Autodesk Inventor part; units mm, degrees
ref_plane "YZ Plane" through (0, 0, 0) normal (1, 0, 0) x (0, 1, 0)
ref_plane "XZ Plane" through (0, 0, 0) normal (0, 1, 0) x (-1, 0, 0)
ref_plane "XY Plane" through (0, 0, 0) normal (0, 0, 1) x (1, 0, 0)
sketch "Sketch1" plane through (0, 0, 0) normal (0, 0, 1) x (1, 0, 0)
  line L0 (-12.7, 25.4) -> (12.7, 25.4)
  line L1 (12.7, 25.4) -> (12.7, -25.4)
  line L2 (12.7, -25.4) -> (-12.7, -25.4)
  line L3 (-12.7, -25.4) -> (-12.7, 25.4)
  line L4 (-12.7, 25.4) -> (12.7, -25.4) construction
  line L5 (12.7, 25.4) -> (-12.7, -25.4) construction
  point P0 (0, 0)
  dimension "d0" = 25.4
  dimension "d1" = 50.8
extrude "Extrusion1" add sketch "Sketch1" along normal blind 1.397
sketch "Sketch3" plane through (12.7, -25.4, 0) normal (1, 0, 0) x (0, 0, -1)
  line L0 (0, 50.8) -> (0, 0)
  line L1 (0, 50.8) -> (-1.397, 50.8)
  line L2 (-1.397, 0) -> (-1.397, 50.8)
  line L3 (0, 0) -> (-1.397, 0)
  line L4 (-1.397, 0) -> (-1.905, 0)
  line L5 (-1.397, 0) -> (-1.397, 1.27)
  line L6 (-1.397, 53.34) -> (-1.397, 0)
  line L7 (-1.651, 1.27) -> (-1.397, 1.27)
  line L8 (-1.651, 1.27) -> (-1.905, 0)
  point P0 (0, 25.4)
  dimension "d8" = 0.508
  dimension "d9" = 1.27
  dimension "d10" = 0.254
ref_plane "Work Plane1" through (0, 0, 1.651) normal (0, 0, 1) x (1, 0, 0)
sketch "Sketch6" plane through (0, 0, 1.651) normal (0, 0, 1) x (1, 0, 0)
  line L0 (12.7, -24.13) -> (12.7, -25.4)
  line L1 (12.7, -25.4) -> (12.7, 25.4)
  line L2 (12.7, -24.765) -> (-12.7, -24.765)
  line L3 (-12.7, -25.4) -> (12.7, -25.4)
  line L4 (-12.7, -25.4) -> (12.7, -25.4)
  point P0 (0, 0)
  dimension "d12" = 0.635
sweep "Sweep1" add profiles "Sketch3" path "Sketch6" path curves L2 contours L4 L8 L7 L2
ref_plane "Work Plane2" through (-12.7, 0, 0) normal (0, -1, 0) x (1, 0, 0)
properties part number "wall"
Design review of the part built by this model. Coordinates are the model's own, in mm. A direction names the side the tool comes from. Coordinates: 2 decimals unless noted, no trailing zeros. Write each loop counter-clockwise with the first axis right and the second up, starting at its lowest first coordinate (ties: lowest second). Pieces come first, ordered by that corner, then holes.
1) Add section B-B (y = -8). Write out the cut boundary in (x, z), plus the area to 3 significant figures.
2) Insertion check: pin 1 (12 mm diameter, centred on x = 5, y = 2.5, fed in from +Z). The pin has a flat end and moves straight along its axis. Give the tip position at first contact, or say it passes through.
3) Machinability: for faces 1 (the flat face through (0, 1, 1.397)), 2 (the flat face through (-12.7, 0, 1)), which of the approach directions +Z, -Z, +X, -X, +Y, -Y give a long, thin tool a straight path to every point of the face, cutting with its end or side? Answer none if there is none.
4) To check wall thickness, follow L1, parallel to Z at x = -11, y = -1.5; L2, parallel to Y at x = 9, z = 1.5. State the ranges of each line that lie inside material, in increasing order.
5) Add section A-A (x = 5.25). Write out the cut boundary in (y, z) (3 decimals), plus the area to 3 significant figures.
Check result:
1. outline: (-12.7, 0) - (12.7, 0) - (12.7, 1.4) - (-12.7, 1.4) - close
1. area: 35.5 mm2
2. pin 1: stops at z = 1.4
3. face 1: +Z, +X, -X, +Y
3. face 2: +Z, -Z, -X, +Y, -Y
4. L1: z = 0 to 1.4
4. L2: y = -25.4 to -24.13
5. outline: (-25.4, 0) - (25.4, 0) - (25.4, 1.397) - (-24.13, 1.397) - (-24.13, 1.651) - (-25.4, 1.905) - close
5. area: 71.5 mm2
